```python
from build123d import *

# Parameters (mm, degrees)
SKETCH1_W                     = 46
SKETCH1_H                     = 11.75
BOSS_EXTRUDE1_DEPTH           = 80
SKETCH2_W                     = 1.2
SKETCH2_H                     = 5.25
BOSS_EXTRUDE2_DEPTH           = 80
SKETCH3_W                     = 40
SKETCH3_H                     = 66
CIRCUIT_BOARD_CLEARANCE_DEPTH = 21
M3X0_5_TAPPED_HOLE1_D         = 2.5
M3X0_5_TAPPED_HOLE2_D         = 2.5
M3X0_5_TAPPED_HOLE2_DEPTH     = 5
M3X0_5_TAPPED_HOLE2_TIP       = 0.751075774
M3X0_5_TAPPED_HOLE3_D         = 2.5


with BuildPart() as part:
    # Sketch1 → Boss-Extrude1 (new body)
    with BuildSketch(Plane(origin=(0, 0, 0), x_dir=(1, 0, 0), z_dir=(0, 1, 0))):
        with Locations((0, 5.875)):
            Rectangle(SKETCH1_W, SKETCH1_H)
    extrude(amount=BOSS_EXTRUDE1_DEPTH)

    # Sketch2 → Boss-Extrude2 (add)
    with BuildSketch(Plane(origin=(0, 0, 0), x_dir=(1, 0, 0), z_dir=(0, 1, 0))):
        with Locations((-22.4, -2.625)):
            Rectangle(SKETCH2_W, SKETCH2_H)
        with Locations((22.4, -2.625)):
            Rectangle(SKETCH2_W, SKETCH2_H)
    extrude(amount=BOSS_EXTRUDE2_DEPTH)

    # Sketch3 → Circuit Board clearance (add)
    with BuildSketch(Plane.XY):
        with Locations((0, 39.7)):
            Rectangle(SKETCH3_W, SKETCH3_H)
    extrude(amount=CIRCUIT_BOARD_CLEARANCE_DEPTH)

    # M3x0.5 Tapped Hole1 (through all)
    with Locations(Plane.XY):
        with Locations((-10, 77), (10, 77), (-10, 3), (10, 3)):
            Hole(M3X0_5_TAPPED_HOLE1_D / 2)

    # M3x0.5 Tapped Hole2
    with Locations(Plane(origin=(0, 80, 0), x_dir=(1, 0, 0), z_dir=(0, 1, 0))):
        with Locations((-15, 2.75), (15, 2.75)):
            Hole(M3X0_5_TAPPED_HOLE2_D / 2, depth=M3X0_5_TAPPED_HOLE2_DEPTH)
            with Locations((0, 0, -(M3X0_5_TAPPED_HOLE2_DEPTH + M3X0_5_TAPPED_HOLE2_TIP / 2))):  # 118° drill point
                Cone(0, M3X0_5_TAPPED_HOLE2_D / 2, M3X0_5_TAPPED_HOLE2_TIP, mode=Mode.SUBTRACT)

    # M3x0.5 Tapped Hole3 (through all)
    with Locations(Plane(origin=(23, 0, 0), x_dir=(0, 0, -1), z_dir=(1, 0, 0))):
        with Locations((3.75, 70), (3.75, 10)):
            Hole(M3X0_5_TAPPED_HOLE3_D / 2)


solid = part.part
```
Could you check a few things on this model? Use its own coordinates, in mm. A direction names the side the tool comes from. Give positions to 0.01 mm unless a question says otherwise; leave off trailing zeros. Loops run counter-clockwise (first coordinate to the right, second up) from the corner with the lowest first, then second, coordinate; pieces in that order, holes last. Notation, with made-up numbers: (83.25, 68.25) - (111.25, 68.25) arc R13 cw to (111.25, 84.25) - close; hole circle Ø9 at (26, -22). An arc over 180 degrees is marked (long way). Use one line per item in the form item = value.
1. I'm going to push flat-ended pins straight in: pin 1 Ø1 at (x, z) = (10, 7) entering from +Y; pin 2 Ø8 at (y, z) = (49.5, 17.5) entering from -X; pin 3 Ø3 at (x, y) = (-10, 3) entering from +Z. Where does each tip first touch, or does it pass through?
Response values:
pin_1 = 72.7
pin_2 = -20
pin_3 = 0
2. I want a section at C-C (y = 3). Please give me the cut outline in (x, z).
Response values:
outline = (-23, -11.75) - (-11.25, -11.75) - (-11.25, 0) - (-21.8, 0) - (-21.8, 5.25) - (-23, 5.25) - close; (-8.75, -11.75) - (8.75, -11.75) - (8.75, 0) - (-8.75, 0) - close; (11.25, -11.75) - (23, -11.75) - (23, 5.25) - (21.8, 5.25) - (21.8, 0) - (11.25, 0) - close
3. I want a section at B-B (x = 1). Please give me the cut outline in (y, z), and give its area (3 significant figures).
Response values:
outline = (0, -11.75) - (80, -11.75) - (80, 0) - (72.7, 0) - (72.7, 21) - (6.7, 21) - (6.7, 0) - (0, 0) - close; hole circle Ø2.5 at (10, -3.75); hole circle Ø2.5 at (70, -3.75)
area = 2,320 mm²
4. I want a section at D-D (y = 70). Please give me the cut outline in (x, z), and give its area (3 significant figures).
Response values:
outline = (-23, -11.75) - (23, -11.75) - (23, -5) - (-23, -5) - close; (-23, -2.5) - (23, -2.5) - (23, 5.25) - (21.8, 5.25) - (21.8, 0) - (20, 0) - (20, 21) - (-20, 21) - (-20, 0) - (-21.8, 0) - (-21.8, 5.25) - (-23, 5.25) - close
area = 1,280 mm²
5. I need wall thicknesses on probe 1 along Y at (x, z) = (-10, -8.75); probe 2 along Y at (x, z) = (13, -3.75); probe 3 along Z at (x, y) = (-15, 78). Which ranges of each line are inside material? Lowest first, please.
Response values:
probe_1 = 0 to 1.75, 4.25 to 75.75, 78.25 to 80
probe_2 = 0 to 8.75, 11.25 to 68.75, 71.25 to 80
probe_3 = -11.75 to -4, -1.5 to 0
6. On a 3-axis mill with a long thin cutter (end or side, diameter ignored), from which of +Z, -Z, +X, -X, +Y, -Y can I reach the whole of each face in a straight line? I mean faces 1 (the face through (-0.32, 11.24, -3.91)), 2 (the face through (-20, 39, 10)), 3 (the face through (16.25, 77.46, -2.8)), 4 (the face through (0, 6.7, 10)). Say none if no direction works.
Response values:
face_1 = +X, -X
face_2 = +Z, +Y, -Y
face_3 = +Y
face_4 = +Z, -Y
7. Thinking about a two-plate mould opening in Z: for faces 5 (the face through (0, 80, -7)), 6 (the face through (-14.079, 77.465, -3.595)), 7 (the face through (0, 40, 21)), which applies, released by +Z, released by -Z, zero draft, split by the parting line, or undercut?
Response values:
face_5 = zero draft
face_6 = undercut
face_7 = released by +Z
8. I want a section at A-A (z = 2). Please give me the cut outline in (x, y).
Response values:
outline = (-23, 0) - (-21.8, 0) - (-21.8, 80) - (-23, 80) - close; (-20, 6.7) - (20, 6.7) - (20, 72.7) - (-20, 72.7) - close; (21.8, 0) - (23, 0) - (23, 80) - (21.8, 80) - close
